The listing builds one solid part. Answer for the finished solid, in the listing's coordinates (mm). A direction names the side the tool comes from. Round coordinates to 2 decimals unless told otherwise and drop trailing zeros. Loops run counter-clockwise (first coordinate to the right, second up) from the corner with the lowest first, then second, coordinate; pieces in that order, holes last. Notation, with made-up numbers: M -25.5,0.5 L 10.5,0.5 A22 ccw 10.5,22.5 Z; hole C -17.5,72.5 d6. An arc over 180 degrees is marked long. Answer as a JSON object with one key per item and string values.
```python
from build123d import *

# Parameters (mm, degrees)
SKETCH1_R           = 2.5
SKETCH1_R_2         = 6
BOSS_EXTRUDE1_DEPTH = 9
SKETCH2_R           = 12.5
SKETCH2_R_2         = 6
BOSS_EXTRUDE2_DEPTH = 4


with BuildPart() as part:
    # Sketch1 → Boss-Extrude1 (new body)
    with BuildSketch(Plane.XY):
        with BuildLine():
            Line((21.365459931, -6), (3, -14))
            Line((3, -14), (-3, -14))
            Line((-3, -14), (-21.365459931, -6))
            ThreePointArc((-21.365459931, -6), (-23.5, 0), (-21.365459931, 6))
            Line((-21.365459931, 6), (-3, 14))
            Line((-3, 14), (3, 14))
            Line((3, 14), (21.365459931, 6))
            ThreePointArc((21.365459931, 6), (23.5, 0), (21.365459931, -6))
        make_face()
        with Locations((-18, 0)):
            Circle(SKETCH1_R, mode=Mode.SUBTRACT)
        with Locations((18, 0)):
            Circle(SKETCH1_R, mode=Mode.SUBTRACT)
        Circle(SKETCH1_R_2, mode=Mode.SUBTRACT)
    extrude(amount=BOSS_EXTRUDE1_DEPTH)

    # Sketch2 → Boss-Extrude2 (add)
    with BuildSketch(Plane.XY.offset(9)):
        Circle(SKETCH2_R)
        Circle(SKETCH2_R_2, mode=Mode.SUBTRACT)
    extrude(amount=BOSS_EXTRUDE2_DEPTH)


solid = part.part
```
Item 1: The part is cut by section B-B (y = 0). Give the vertices of the cut face in (x, z).
Values follow:
{"outline": "M -23.5,0 L -20.5,0 L -20.5,9 L -23.5,9 Z; M -15.5,0 L -6,0 L -6,13 L -12.5,13 L -12.5,9 L -15.5,9 Z; M 6,0 L 15.5,0 L 15.5,9 L 12.5,9 L 12.5,13 L 6,13 Z; M 20.5,0 L 23.5,0 L 23.5,9 L 20.5,9 Z"}
Item 2: Which of the six approach directions +Z, -Z, +X, -X, +Y, -Y give full straight-line access (tool end or side, diameter ignored) to faces 1 (the face through (-2, 13, 9)), 2 (the face through (23.5, 0.1, 4.4))?
Values follow:
{"face 1": "+Z", "face 2": "+Z, -Z, +X"}
Item 3: Determine the mould class of faces 3 (the face through (-20.5, 0.1, 4.4)), 4 (the face through (-12.054, -10.056, 4.437)), 5 (the face through (12.054, 10.056, 4.437)) for opening direction Y: released by +Y, released by -Y, zero draft, split by the parting line, or undercut.
Values follow:
{"face 3": "undercut", "face 4": "released by -Y", "face 5": "released by +Y"}
Item 4: The part is cut by section A-A (x = 0). Give the vertices of the cut face in (y, z), then the cut area to 3 significant figures.
Values follow:
{"outline": "M -14,0 L -6,0 L -6,13 L -12.5,13 L -12.5,9 L -14,9 Z; M 6,0 L 14,0 L 14,9 L 12.5,9 L 12.5,13 L 6,13 Z", "area": "196 mm^2"}
Item 5: Flat-ended cylindrical pins translate along their axes: P1, Ø1.5, axis at x = -15, z = 3, coming from the -Y side; P2, Ø4, axis at y = -9, z = 2, coming from the +X side; P3, Ø1.5, axis at x = -16.5, z = 4.5, coming from the +Y side. Find the tip coordinate at first contact, or state that the pin passes through.
Values follow:
{"P1": "y = -9.1", "P2": "x = 19.07", "P3": "y = 8.45"}
Item 6: The part is cut by section D-D (z = 10.5). Give the vertices of the cut face in (x, y), then the cut area to 3 significant figures.
Values follow:
{"outline": "C 0,0 d25; hole C 0,0 d12", "area": "378 mm^2"}
Item 7: The part is cut by section C-C (y = 5.25). Give the vertices of the cut face in (x, z), then the cut area to 3 significant figures.
Values follow:
{"outline": "M -21.92,0 L -2.9,0 L -2.9,13 L -11.34,13 L -11.34,9 L -21.92,9 Z; M 2.9,0 L 21.92,0 L 21.92,9 L 11.34,9 L 11.34,13 L 2.9,13 Z", "area": "410 mm^2"}
Item 8: Straight lines are drawn through the part: line 1 (X direction, y = 2, z = 5.25); line 2 (Y direction, x = 0, z = 3.25); line 3 (X direction, y = 4.5, z = 6.75). For each, find the intervals that lie inside material, in ascending order.
Values follow:
{"line 1": "-23.29 to -19.5, -16.5 to -5.66, 5.66 to 16.5, 19.5 to 23.29", "line 2": "-14 to -6, 6 to 14", "line 3": "-22.37 to -3.97, 3.97 to 22.37"}
